```python
from build123d import *

# Parameters (mm, degrees)
BOSS_EXTRUDE1_DEPTH = 1
BOSS_EXTRUDE2_DEPTH = 1


with BuildPart() as part:
    # Sketch1 → Boss-Extrude1 (new body)
    with BuildSketch(Plane(origin=(0, 0, 0), x_dir=(1, 0, 0), z_dir=(0, 1, 0))):
        Polygon((-17.101249567, 62.026712282), (-17.101249567, 42.026712282), (-44.119439114, 42.026712282), (-44.119439114, 17.026712282), (-4.760262303, -28.259656537), (35.313890805, 16.395267634), (35.313890805, 42.026712282), (8.862371339, 42.026712282), (8.862371339, 62.026712282), align=None)
    extrude(amount=BOSS_EXTRUDE1_DEPTH)

    # Sketch2 → Boss-Extrude2 (add)
    with BuildSketch(Plane(origin=(0, 1, 0), x_dir=(1, 0, 0), z_dir=(0, 1, 0))):
        Polygon((8.862371339, -28.259656537), (-17.101249567, -28.259656537), (-17.101249567, 42.026712282), (8.862371339, 62.026712282), align=None)
    extrude(amount=-BOSS_EXTRUDE2_DEPTH)


solid = part.part
```
CAD build for the part. Positions are in the model's coordinates, mm. Round coordinates to 2 decimals unless told otherwise and drop trailing zeros. Order: outer loops, then holes, each group sorted by start corner. A loop starts at its lowest first (then second) coordinate and runs counter-clockwise, first axis right, second up. Notation, with made-up numbers: (52, 40.5) - (61, 40.5) arc R21 ccw to (61, 56.5) - close; hole circle Ø2 at (6.5, 82). An arc over 180 degrees is marked (long way). Answer in a Markdown table with one row per item. Add a question column.
(1) Band-saw the part on B-B on z = 21. List the corners of the cut face in (x, y), and give its area (3 significant figures).
(2) Band-saw the part on C-C on x = -33. List the corners of the cut face in (y, z), and give its area (3 significant figures).
(3) Drop a flat-ended pin along its axis: pin 1 Ø0.5 at (x, y) = (-29, 0.5) entering from -Z. Give the stop position or say it passes through.
(4) Band-saw the part on A-A on y = 0.45. List the corners of the cut face in (x, z).
(5) Probe L1, parallel to X at y = 0.55, z = -48.5; L2, parallel to Z at x = -34, y = 0.35; L3, parallel to Z at x = -37.5, y = 0.35. List the from-to ranges inside material, lowest first. Write a range as [from, to].
Data:
| question | item | result |
|---|---|---|
| 1 | outline | (-17.1, 0) - (8.86, 0) - (8.86, 1) - (-17.1, 1) - close |
| 1 | area | 26.0 mm^2 |
| 2 | outline | (0, -42.03) - (1, -42.03) - (1, -4.23) - (0, -4.23) - close |
| 2 | area | 37.8 mm^2 |
| 3 | pin 1 | stops at z = -42.03 |
| 4 | outline | (-44.12, -42.03) - (-17.1, -42.03) - (-17.1, -62.03) - (8.86, -62.03) - (8.86, -42.03) - (35.31, -42.03) - (35.31, -16.4) - (8.86, 13.08) - (8.86, 28.26) - (-17.1, 28.26) - (-17.1, 14.06) - (-44.12, -17.03) - close |
| 5 | L1 | x = [-17.1, 8.86] |
| 5 | L2 | z = [-42.03, -5.38] |
| 5 | L3 | z = [-42.03, -9.41] |
